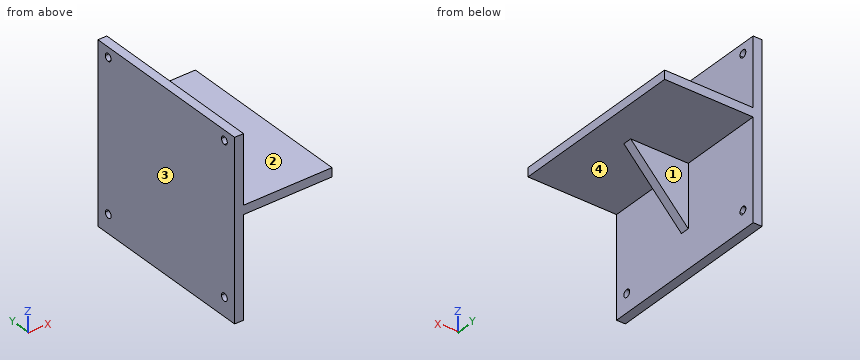
```python
from build123d import *

# Parameters (mm, degrees)
F1_DEPTH = 200
F2_W     = 10
F2_H     = 70
F3_DEPTH = 70
F5_DEPTH = 100
F6_DEPTH = 75.001


with BuildPart() as f1:
    # F0 (on Front) → F1 (new body)
    with BuildSketch(Plane.XZ):
        Polygon((5, 100), (-5, 100), (-5, 23.2), (-5, 13.2), (-5, -100), (5, -100), (5, 13.2), (105, 13.2), (105, 23.2), (5, 23.2), align=None)
    extrude(amount=F1_DEPTH)

    # F2 (on Right) → F3 (join)
    with BuildSketch(Plane.YZ):
        with Locations((-100, -21.8)):
            Rectangle(F2_W, F2_H)
        with BuildLine():
            Line((-185, 84.6313585043), (-185, 88.8813585043))
            Line((-185, 88.8813585043), (-180.75, 88.8813585043))
            ThreePointArc((-180.75, 88.8813585043), (-188.00520382, 91.8865623243), (-185, 84.6313585043))
        make_face()
        with BuildLine():
            Line((-180.75, 88.8813585043), (-185, 88.8813585043))
            Line((-185, 88.8813585043), (-185, 84.6313585043))
            ThreePointArc((-185, 84.6313585043), (-181.99479618, 85.8761546843), (-180.75, 88.8813585043))
        make_face()
        with BuildLine():
            Line((-185, -74.8090941906), (-185, -79.0590941906))
            Line((-185, -79.0590941906), (-180.75, -79.0590941906))
            ThreePointArc((-180.75, -79.0590941906), (-181.99479618, -76.0538903706), (-185, -74.8090941906))
        make_face()
        with BuildLine():
            Line((-180.75, -79.0590941906), (-185, -79.0590941906))
            Line((-185, -79.0590941906), (-185, -74.8090941906))
            ThreePointArc((-185, -74.8090941906), (-188.00520382, -82.0642980106), (-180.75, -79.0590941906))
        make_face()
        with BuildLine():
            Line((-19.25, -79.0590941906), (-15, -79.0590941906))
            Line((-15, -79.0590941906), (-15, -74.8090941906))
            ThreePointArc((-15, -74.8090941906), (-18.00520382, -76.0538903706), (-19.25, -79.0590941906))
        make_face()
        with BuildLine():
            Line((-15, -74.8090941906), (-15, -79.0590941906))
            Line((-15, -79.0590941906), (-19.25, -79.0590941906))
            ThreePointArc((-19.25, -79.0590941906), (-15, -83.3090941906), (-10.75, -79.0590941906))
            ThreePointArc((-10.75, -79.0590941906), (-11.99479618, -76.0538903706), (-15, -74.8090941906))
        make_face()
        with BuildLine():
            ThreePointArc((-15, 84.6313585043), (-11.99479618, 85.8761546843), (-10.75, 88.8813585043))
            ThreePointArc((-10.75, 88.8813585043), (-15, 93.1313585043), (-19.25, 88.8813585043))
            Line((-19.25, 88.8813585043), (-15, 88.8813585043))
            Line((-15, 88.8813585043), (-15, 84.6313585043))
        make_face()
        with BuildLine():
            Line((-15, 88.8813585043), (-19.25, 88.8813585043))
            ThreePointArc((-19.25, 88.8813585043), (-18.00520382, 85.8761546843), (-15, 84.6313585043))
            Line((-15, 84.6313585043), (-15, 88.8813585043))
        make_face()
    extrude(amount=F3_DEPTH)

    # F4 (on face) → F5 (cut)
    with BuildSketch(Plane.XZ.offset(105)):
        Polygon((5, -56.8), (70, -56.8), (70, 13.2), align=None)
    extrude(amount=-F5_DEPTH, mode=Mode.SUBTRACT)

    # F6 (cut, through all): faces of the model
    f6_faces = [f1.faces().sort_by_distance(p)[0] for p in [
        (70, -185, 88.8813585043),
        (70, -15, 88.8813585043),
        (70, -15, -79.0590941906),
        (70, -185, -79.0590941906),
    ]]
    extrude(f6_faces, amount=-F6_DEPTH, mode=Mode.SUBTRACT)


solid = f1.part
```
Verification items for the finished model (mm, model axes). Face numbers are marked on the shaded views. A direction names the side the tool comes from. Coordinates: 2 decimals unless noted, no trailing zeros. Loops run counter-clockwise (first coordinate to the right, second up) from the corner with the lowest first, then second, coordinate; pieces in that order, holes last. Notation, with made-up numbers: (51, 58.25) - (108, 58.25) arc R12 ccw to (108, 63.25) - close; hole circle Ø11 at (34, 4.5). An arc over 180 degrees is marked (long way). Answer as a JSON object with one key per item and string values.
(1) Cross-section at A-A, the plane y = -66.5. Record the boundary of the cut face in (x, z), then the cut area to 3 significant figures.
Response:
{"outline": "(-5, -100) - (5, -100) - (5, 13.2) - (105, 13.2) - (105, 23.2) - (5, 23.2) - (5, 100) - (-5, 100) - close", "area": "3,000 mm²"}
(2) Access from +Z, -Z, +X, -X, +Y, -Y to the whole of each face (thin tool, end or side, straight path). Record for the marked faces 1, 2, 3 and 4.
Response:
{"face 1": "-Z, +X, +Y", "face 2": "+Z, +X, +Y, -Y", "face 3": "+Z, -Z, -X, +Y, -Y", "face 4": "-Z, +X"}
(3) Cross-section at D-D, the plane x = 87. Record the boundary of the cut face in (y, z).
Response:
{"outline": "(-200, 13.2) - (0, 13.2) - (0, 23.2) - (-200, 23.2) - close"}
(4) Cross-section at B-B, the plane x = 48. Record the boundary of the cut face in (y, z).
Response:
{"outline": "(-200, 13.2) - (-105, 13.2) - (-105, -10.49) - (-95, -10.49) - (-95, 13.2) - (0, 13.2) - (0, 23.2) - (-200, 23.2) - close"}
(5) Go/stop test with flat-tipped pins: pin 1 Ø11 at (y, z) = (-185, -79.06) entering from +X; pin 2 Ø3 at (x, y) = (31, -33.5) entering from -Z; pin 3 Ø12 at (x, z) = (53.5, -11.5) entering from -Y; pin 4 Ø13.5 at (y, z) = (-185, 88.88) entering from -X. Record where each tip stops, or that it passes through.
Response:
{"pin 1": "stops at x = 5", "pin 2": "stops at z = 13.2", "pin 3": "stops at y = -105", "pin 4": "stops at x = -5"}
(6) Scan lines: line 1 along Z through (x, y) = (-1.5, -185); line 2 along Z through (x, y) = (18, -160); line 3 along X through (y, z) = (-122, -89.5). Record each from-to range of solid material in increasing order.
Response:
{"line 1": "z = -100 to -83.31, -74.81 to 84.63, 93.13 to 100", "line 2": "z = 13.2 to 23.2", "line 3": "x = -5 to 5"}
(7) Cross-section at C-C, the plane z = -64. Record the boundary of the cut face in (x, y), then the cut area to 3 significant figures.
Response:
{"outline": "(-5, -200) - (5, -200) - (5, 0) - (-5, 0) - close", "area": "2,000 mm²"}
